Geometry check sheet. Reference: the model listing, model coordinates, mm. Face numbers are marked on the shaded views. Give positions to 0.01 mm unless a question says otherwise; leave off trailing zeros. Order: outer loops, then holes, each group sorted by start corner. A loop starts at its lowest first (then second) coordinate and runs counter-clockwise, first axis right, second up.
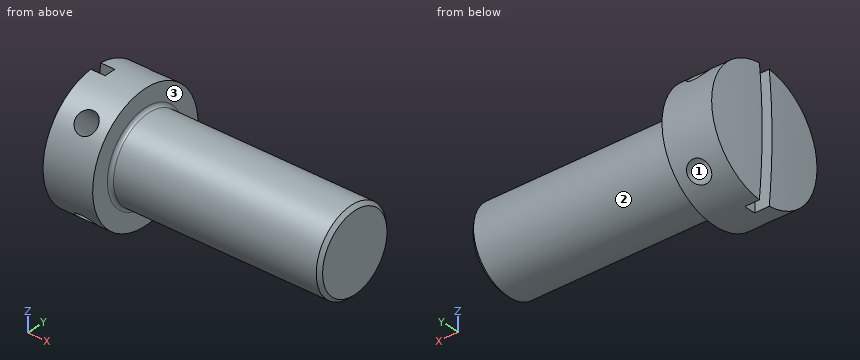
from build123d import *

# Parameters (mm, degrees)
FILLET1_R         = 0.8
SLOT_DEPTH        = 67.001893912
SLOT_DEPTH_BACK   = 67.001893912
HOLESKE_R         = 2.59
DRILL_HOLE_DEPTH  = 67.001893912
DRILL_HOLES_COUNT = 2
DRILL_HOLES_ANGLE = 90


with BuildPart() as part:
    # BodySke → Base-Revolve (revolve)
    with BuildSketch(Plane.XY, mode=Mode.PRIVATE) as base_revolve_sk:
        with BuildLine():
            Line((0.65, 15), (12.5, 15))
            Line((12.5, 15), (12.5, 10))
            Line((12.5, 10), (61.672, 10))
            Line((61.672, 10), (62.5, 9.172))
            Line((62.5, 9.172), (62.5, 0))
            Line((62.5, 0), (0, 0))
            ThreePointArc((0, 0), (0.162576213, 7.507038364), (0.65, 15))
        make_face()
    revolve(base_revolve_sk.sketch.rotate(Axis((-31.75, 0, 0), (1, 0, 0)), 90), axis=Axis((-31.75, 0, 0), (1, 0, 0)))

    # Fillet1
    fillet1_edges = [part.edges().sort_by_distance(p)[0] for p in [
        (12.5, 0, -10),
    ]]
    fillet(fillet1_edges, radius=FILLET1_R)

    # Sketch3 → Slot (cut, two sides: drawn at the far end of the back side and taken through both)
    with BuildSketch(Plane.XY.offset(-SLOT_DEPTH_BACK)):
        Polygon((-139.217564887, 1.405), (0.005692144, 1.405), (4.105692144, 1.405), (4.105692144, -1.405), (0.005692144, -1.405), (-139.217564887, -1.405), (-417.664078948, -1.405), (-417.664078948, 1.405), align=None)
    extrude(amount=SLOT_DEPTH + SLOT_DEPTH_BACK, mode=Mode.SUBTRACT)

    # HoleSke → Drill Hole (cut, symmetric)
    with BuildSketch(Plane(origin=(0, 0, 0), x_dir=(1, 0, 0), z_dir=(0, 0.7071067811865462, 0.7071067811865488))):
        with Locations(Location((7.35, 0, 0), (0, 0, 270))):
            Circle(HOLESKE_R)
    drill_hole = extrude(amount=DRILL_HOLE_DEPTH, both=True, mode=Mode.SUBTRACT)

    # Drill Holes: Drill Hole ×2 about axis
    drill_holes_axis = Axis((0, 0, 0), (1, 0, 0))
    for i in range(1, DRILL_HOLES_COUNT):
        add(drill_hole.rotate(drill_holes_axis, i * DRILL_HOLES_ANGLE / (DRILL_HOLES_COUNT - 1)), mode=Mode.SUBTRACT)


solid = part.part
Item 1: Scan lines: L1, parallel to Y at x = 9, z = -7.5; L2, parallel to Z at x = 50.5, y = 0.5; L3, parallel to X at y = 7, z = -5.5. Record each from-to range of solid material in increasing order.
Reported:
L1: y = -12.99 to -10.32, -4.68 to 4.68, 10.32 to 12.99
L2: z = -9.99 to 9.99
L3: x = 0.23 to 4.99, 9.71 to 62.5
Item 2: Sectioned sample at B-B (x = 14). Enter the section's corners in (y, z).
Reported:
outline: circle Ø20 at (0, 0)
Item 3: Draft check along X on the marked faces 1, 2 and 3. Enter one of: released by +X, released by -X, zero draft, split by the parting line, or undercut.
Reported:
face 1: undercut
face 2: zero draft
face 3: released by +X
Item 4: Gauge pin test, flat ends, axial feed: pin 1 (10 mm diameter, centred on x = 54.5, z = 5, fed in from +Y); pin 2 (2 mm diameter, centred on x = 1.5, z = 5, fed in from +Y); pin 3 (6 mm diameter, centred on x = 14.5, z = -9, fed in from -Y). Record the tip position at first contact, or that the pin passes through.
Reported:
pin 1: stops at y = 10
pin 2: stops at y = 14.46
pin 3: stops at y = -13.39
Item 5: Sectioned sample at C-C (y = 13). Enter the section's corners in (x, z).
Reported:
outline: (0.65, -7.48) - (12.5, -7.48) - (12.5, 7.48) - (0.65, 7.48) arc R172.91 ccw to start
Item 6: Sectioned sample at A-A (z = -6). Give the number of separate pieces and of enclosed holes in the cut face, and give its area (3 significant figures).
Reported:
separate pieces: 1
enclosed holes: 2
area: 1,060 mm2
